Can you work these out from the model? Positions are in its coordinate system, mm. A direction names the side the tool comes from. Give positions to 0.01 mm unless a question says otherwise; leave off trailing zeros. Order: outer loops, then holes, each group sorted by start corner. A loop starts at its lowest first (then second) coordinate and runs counter-clockwise, first axis right, second up. Notation, with made-up numbers: (69.5, -21) - (88.5, -21) arc R34 cw to (88.5, 13) - close; hole circle Ø2 at (4, 37). An arc over 180 degrees is marked (long way). Answer as CSV lines item,"result".
Autodesk Inventor part; units mm, degrees
ref_plane "YZ Plane" through (0, 0, 0) normal (1, 0, 0) x (0, 1, 0)
ref_plane "XZ Plane" through (0, 0, 0) normal (0, 1, 0) x (-1, 0, 0)
ref_plane "XY Plane" through (0, 0, 0) normal (0, 0, 1) x (1, 0, 0)
sketch "Sketch1" plane through (0, 0, 0) normal (1, 0, 0) x (0, 1, 0)
  line L0 (0.0055, 3.1659) -> (2.7555, 1.5782)
  line L1 (2.7555, 1.5782) -> (2.7555, -1.5973)
  line L2 (2.7555, -1.5973) -> (0.0055, -3.185)
  line L3 (0.0055, -3.185) -> (-2.7445, -1.5973)
  line L4 (-2.7445, -1.5973) -> (-2.7445, 1.5782)
  line L5 (-2.7445, 1.5782) -> (0.0055, 3.1659)
  point P0 (0.0055, -0.0095)
  dimension "d1" = 5.5
extrude "Extrusion1" add sketch "Sketch1" along normal blind 11.5
sketch "Sketch2" plane through (0, 0, 0) normal (-1, 0, 0) x (0, 0, 1)
  circle A0 centre (0, 0) radius 1.5
  dimension "d4" = 3
extrude "Extrusion2" add sketch "Sketch2" along normal blind 4
sketch "Sketch3" plane through (11.5, 0, 0) normal (1, 0, 0) x (0, 0, -1)
  circle A0 centre (0, 0) radius 1.5
  dimension "d7" = 3
extrude "Extrusion3" cut sketch "Sketch3" against normal blind 6.018
properties part number "Spacer"
1) I want a section at D-D on z = 0. Write out the boundary of the cut face in (x, y), plus the area to 3 significant figures.
Answer block:
outline,"(-4, -1.5) - (0, -1.5) - (0, -2.74) - (11.5, -2.74) - (11.5, -1.5) - (5.48, -1.5) - (5.48, 1.5) - (11.5, 1.5) - (11.5, 2.76) - (0, 2.76) - (0, 1.5) - (-4, 1.5) - close"
area,"57.2 mm2"
2) I'm going to push flat-ended pins straight in: P1, Ø0.9, axis at y = 0, z = -0.5, coming from the +X side; P2, Ø2, axis at x = 0.5, y = 2, coming from the +Z side. Where does each tip first touch, or does it pass through?
Answer block:
P1,"x = 5.48"
P2,"z = 2.59"
3) I want a section at C-C on x = 1.5. Write out the boundary of the cut face in (y, z) (1 decimal), plus the area to 3 significant figures.
Answer block:
outline,"(-2.7, -1.6) - (0, -3.2) - (2.8, -1.6) - (2.8, 1.6) - (0, 3.2) - (-2.7, 1.6) - close"
area,"26.2 mm2"
4) I want a section at A-A on x = 9.75. Write out the boundary of the cut face in (y, z) (1 decimal).
Answer block:
outline,"(-2.7, -1.6) - (0, -3.2) - (2.8, -1.6) - (2.8, 1.6) - (0, 3.2) - (-2.7, 1.6) - close; hole circle Ø3 at (0, 0)"
5) If we mould it in two halves opening along Z, with no side actions, what happens to faces 1 (the flat face through (5.482, 0, 0)), 2 (the cylindrical face through (8.53, 0.07, 1.5)), 3 (the flat face through (5.67, 1.4, -2.38)), 4 (the cylindrical face through (-1.97, -0.07, -1.5))? For each: +Z half, -Z half, draft (parallel to the pull), parting line (faces both ways), or undercut.
Answer block:
face 1,"undercut"
face 2,"undercut"
face 3,"-Z half"
face 4,"parting line"
6) I need wall thicknesses on line 1 along Y through (x, z) = (7, 0); line 2 along X through (y, z) = (-1.05, 0.5); line 3 along X through (y, z) = (-1.3, 1.75). Which ranges of each line are inside material? Lowest first, please. Write a range as [from, to].
Answer block:
line 1,"[-2.74, -1.5], [1.5, 2.76]"
line 2,"[-4, 5.48]"
line 3,"[0, 11.5]"
7) Which directions (+Z, -Z, +X, -X, +Y, -Y) give clear straight access to the entire face, cutting with the end or side of a thin tool? Please do faces 5 (the flat face through (5.67, -1.39, 2.36)), 6 (the flat face through (0, -1.3, -1.4)).
Answer block:
face 5,"+Z, +X, -X, -Y"
face 6,"-X"
8) I want a section at B-B on y = 1.3. Write out the boundary of the cut face in (x, z), plus the area to 3 significant figures.
Answer block:
outline,"(-4, -0.75) - (0, -0.75) - (0, -2.44) - (11.5, -2.44) - (11.5, -0.75) - (5.48, -0.75) - (5.48, 0.75) - (11.5, 0.75) - (11.5, 2.42) - (0, 2.42) - (0, 0.75) - (-4, 0.75) - close"
area,"52.8 mm2"
